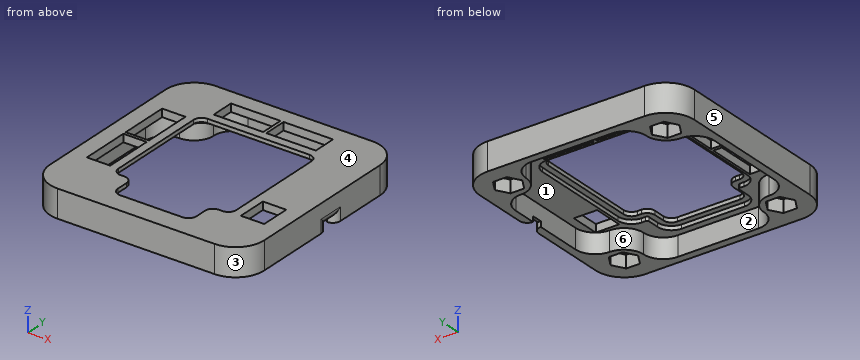
from build123d import *

# Parameters (mm, degrees)
WALL_EXTRUDE_BOSS_START          = 8.64
WALL_EXTRUDE_BOSS_DEPTH          = 7.05
CEILING_EXTRUDE_BOSS_DEPTH       = 2
SCREWS_BLOCKS_EXTRUDE_BOSS_DEPTH = 5.05
SCREWS_BLOCKS_FILLET_R           = 5
NUTS_EXTRUDE_DEPTH               = 3.2
SCREWS_SKETCH_R                  = 2.15
SCREWS_HOOLES_EXTRUDE_DEPTH      = 2.5
CONNECTORS_SKETCH_W              = 12.6
CONNECTORS_SKETCH_H              = 5.95
CONNECTORS_SKETCH_W_2            = 5.95
CONNECTORS_SKETCH_H_2            = 12.6
CONNECTORS_SKETCH_H_3            = 7.6
CONNECTORS_EXTRUDE_DEPTH         = 2.5
SWITCH_SKETCH_W                  = 1.4
SWITCH_SKETCH_H                  = 2.68
SWITCH_EXTRUDE_DEPTH             = 2.5
SWITCH_FILLET_R                  = 2
GLASS_EXTRUDE_DEPTH              = 2.5
GLASS_FIT_EXTRUDE_DEPTH          = 1


with BuildPart() as part:
    # Wall_Sketch → Wall_Extrude_Boss (new body)
    with BuildSketch(Plane.XY.offset(WALL_EXTRUDE_BOSS_START)):
        with BuildLine():
            Line((-52.3, 44.999999897), (-52.29999, 5.00000605))
            ThreePointArc((-52.29999, 5.00000605), (-50.161874571, -0.161870293), (-45, -2.29999))
            Line((-45, -2.29999), (-5.000000575, -2.3))
            ThreePointArc((-5.000000575, -2.3), (0.161879299, -0.161879706), (2.3, 5))
            Line((2.3, 5), (2.3, 45))
            ThreePointArc((2.3, 45), (0.161879503, 50.161879503), (-5, 52.3))
            Line((-5, 52.3), (-45, 52.3))
            ThreePointArc((-45, 52.3), (-50.161879539, 50.161879466), (-52.3, 44.999999897))
        make_face()
        with BuildLine():
            Line((-5, 50.3), (-45, 50.3))
            ThreePointArc((-45, 50.3), (-48.747665967, 48.747665914), (-50.3, 44.999999925))
            Line((-50.3, 44.999999925), (-50.29999, 5.00000655))
            ThreePointArc((-50.29999, 5.00000655), (-48.747661185, 1.252343447), (-45, -0.29999))
            Line((-45, -0.29999), (-5.000000075, -0.3))
            ThreePointArc((-5.000000075, -0.3), (-1.252334086, 1.252334033), (0.3, 5))
            Line((0.3, 5), (0.3, 45))
            ThreePointArc((0.3, 45), (-1.25233406, 48.74766594), (-5, 50.3))
        make_face(mode=Mode.SUBTRACT)
    extrude(amount=-WALL_EXTRUDE_BOSS_DEPTH)

    # Ceiling_Sketch → Ceiling_Extrude_Boss (add)
    with BuildSketch(Plane.XY.offset(8.64)):
        with BuildLine():
            Line((-45, -0.29999), (-5.000000075, -0.3))
            ThreePointArc((-5.000000075, -0.3), (-1.252334086, 1.252334033), (0.3, 5))
            Line((0.3, 5), (0.3, 45))
            ThreePointArc((0.3, 45), (-1.25233406, 48.74766594), (-5, 50.3))
            Line((-5, 50.3), (-45, 50.3))
            ThreePointArc((-45, 50.3), (-48.747665967, 48.747665914), (-50.3, 44.999999925))
            Line((-50.3, 44.999999925), (-50.29999, 5.00000655))
            ThreePointArc((-50.29999, 5.00000655), (-48.747661185, 1.252343447), (-45, -0.29999))
        make_face()
    extrude(amount=-CEILING_EXTRUDE_BOSS_DEPTH)


with BuildPart() as screws_blocks_extrude_boss_tool:
    # Screws_Blocks_Sketch → Screws_Blocks_Extrude_Boss (new body)
    with BuildSketch(Plane(origin=(0, 0, 6.64), x_dir=(-1, 0, 0), z_dir=(0, 0, -1))):
        with BuildLine():
            Line((9.7, -0.299998825), (4.7, -0.299998825))
            ThreePointArc((4.7, -0.299998825), (1.164466094, 1.164467269), (-0.3, 4.700001175))
            Line((-0.3, 4.700001175), (-0.3, 9.700001175))
            Line((-0.3, 9.700001175), (9.7, 9.700001175))
            Line((9.7, 9.700001175), (9.7, -0.299998825))
        make_face()
        with BuildLine():
            Line((9.7, 50.3), (4.7, 50.3))
            ThreePointArc((4.7, 50.3), (1.164466094, 48.835533906), (-0.3, 45.3))
            Line((-0.3, 45.3), (-0.3, 40.3))
            Line((-0.3, 40.3), (9.7, 40.3))
            Line((9.7, 40.3), (9.7, 50.3))
        make_face()
        with BuildLine():
            Line((40.299998825, 50.3), (45.299998825, 50.3))
            ThreePointArc((45.299998825, 50.3), (48.835532731, 48.835533906), (50.299998825, 45.3))
            Line((50.299998825, 45.3), (50.299998825, 40.3))
            Line((50.299998825, 40.3), (40.299998825, 40.3))
            Line((40.299998825, 40.3), (40.299998825, 50.3))
        make_face()
        with BuildLine():
            Line((40.299991175, -0.299991175), (45.299991175, -0.299991175))
            ThreePointArc((45.299991175, -0.299991175), (48.835525081, 1.164474919), (50.299991175, 4.700008825))
            Line((50.299991175, 4.700008825), (50.299991175, 9.700008825))
            Line((50.299991175, 9.700008825), (40.299991175, 9.700008825))
            Line((40.299991175, 9.700008825), (40.299991175, -0.299991175))
        make_face()
    extrude(amount=SCREWS_BLOCKS_EXTRUDE_BOSS_DEPTH)


with BuildPart() as part_1:
    add(part.part)


with BuildPart() as part_2:
    # Screws_Blocks_Extrude_Boss: joined with screws_blocks_extrude_boss_tool
    add(part_1.part.fuse(screws_blocks_extrude_boss_tool.part, tol=0.00001))

    # Screws_Blocks_Fillet
    screws_blocks_fillet_edges = [part_2.edges().sort_by_distance(p)[0] for p in [
        (-40.299998825, 50.3, 4.115),
        (-50.299998825, 40.3, 4.115),
        (-40.299998825, 40.3, 4.115),
        (-9.7, 50.3, 4.115),
        (-9.7, 40.3, 4.115),
        (0.3, 40.3, 4.115),
        (0.3, 9.700001175, 4.115),
        (-9.7, 9.700001175, 4.115),
        (-9.7, -0.299998825, 4.115),
        (-40.299991175, -0.299991175, 4.115),
        (-40.299991175, 9.700008825, 4.115),
        (-50.299991175, 9.700008825, 4.115),
    ]]
    fillet(screws_blocks_fillet_edges, radius=SCREWS_BLOCKS_FILLET_R - 0.0001)  # a hair under: the kernel refuses the full size

    # Nuts_Sketch → Nuts_Extrude (cut)
    with BuildSketch(Plane(origin=(0, 0, 1.59), x_dir=(-1, 0, 0), z_dir=(0, 0, -1))):
        Polygon((1.500002453, 44.995856332), (3.253589748, 41.966841377), (6.753587296, 41.970985045), (8.499997547, 45.004143668), (6.746410252, 48.033158623), (3.246412704, 48.029014955), align=None)
        Polygon((41.5, 45), (43.25, 41.968911087), (46.75, 41.968911087), (48.5, 45), (46.75, 48.031088913), (43.25, 48.031088913), align=None)
        Polygon((41.5, 5), (43.25, 1.968911087), (46.75, 1.968911087), (48.5, 5), (46.75, 8.031088913), (43.25, 8.031088913), align=None)
        Polygon((8.49998026, 4.988245077), (6.760170192, 8.025194356), (3.260189932, 8.03694928), (1.50001974, 5.011754923), (3.239829808, 1.974805644), (6.739810068, 1.96305072), align=None)
    extrude(amount=-NUTS_EXTRUDE_DEPTH, mode=Mode.SUBTRACT)

    # Screws_Sketch → Screws_Hooles_Extrude (cut)
    with BuildSketch(Plane(origin=(0, 0, 4.79), x_dir=(-1, 0, 0), z_dir=(0, 0, -1))):
        with Locations((5, 45)):
            Circle(SCREWS_SKETCH_R)
        with Locations((45, 45)):
            Circle(SCREWS_SKETCH_R)
        with Locations((45, 5)):
            Circle(SCREWS_SKETCH_R)
        with Locations((5, 5)):
            Circle(SCREWS_SKETCH_R)
    extrude(amount=-SCREWS_HOOLES_EXTRUDE_DEPTH, mode=Mode.SUBTRACT)

    # Connectors_Sketch → Connectors_Extrude (cut)
    with BuildSketch(Plane.XY.offset(8.64)):
        with Locations((-31.7, 45.175)):
            Rectangle(CONNECTORS_SKETCH_W, CONNECTORS_SKETCH_H)
        with Locations((-18.3, 45.175)):
            Rectangle(CONNECTORS_SKETCH_W, CONNECTORS_SKETCH_H)
        with Locations((-45.075, 31.7)):
            Rectangle(CONNECTORS_SKETCH_W_2, CONNECTORS_SKETCH_H_2)
        with Locations((-45.075, 18.3)):
            Rectangle(CONNECTORS_SKETCH_W_2, CONNECTORS_SKETCH_H_2)
        with Locations((-4.825, 14.4)):
            Rectangle(CONNECTORS_SKETCH_W_2, CONNECTORS_SKETCH_H_3)
    extrude(amount=-CONNECTORS_EXTRUDE_DEPTH, mode=Mode.SUBTRACT)

    # Switch_Sketch → Switch_Extrude (cut)
    with BuildSketch(Plane(origin=(2.3, 0, 0), x_dir=(0, 0, -1), z_dir=(1, 0, 0))):
        with Locations((-2.24, 28.01)):
            Rectangle(SWITCH_SKETCH_W, SWITCH_SKETCH_H)
    extrude(amount=-SWITCH_EXTRUDE_DEPTH, mode=Mode.SUBTRACT)

    # Switch_Fillet
    switch_fillet_edges = [part_2.edges().sort_by_distance(p)[0] for p in [
        (2.3, 28.01, 2.94),
        (2.3, 29.35, 2.265),
        (2.3, 26.67, 2.265),
    ]]
    fillet(switch_fillet_edges, radius=SWITCH_FILLET_R - 0.0001)  # a hair under: the kernel refuses the full size

    # Glass_Sketch → Glass_Extrude (cut)
    with BuildSketch(Plane(origin=(0, 0, 6.64), x_dir=(-1, 0, 0), z_dir=(0, 0, -1))):
        with BuildLine():
            Line((34.9999975, 8), (34.9999975, 5))
            ThreePointArc((34.9999975, 5), (34.414211062, 3.585786438), (32.9999975, 3))
            Line((32.9999975, 3), (16.9999975, 3))
            ThreePointArc((16.9999975, 3), (15.585783938, 3.585786438), (14.9999975, 5))
            Line((14.9999975, 5), (14.9999975, 8))
            ThreePointArc((14.9999975, 8), (14.414211062, 9.414213562), (12.9999975, 10))
            Line((12.9999975, 10), (11.9999975, 10))
            ThreePointArc((11.9999975, 10), (10.585783938, 10.585786438), (9.9999975, 12))
            Line((9.9999975, 12), (9.9999975, 38))
            ThreePointArc((9.9999975, 38), (10.585783938, 39.414213562), (11.9999975, 40))
            Line((11.9999975, 40), (37.9999975, 40))
            ThreePointArc((37.9999975, 40), (39.414211062, 39.414213562), (39.9999975, 38))
            Line((39.9999975, 38), (39.9999975, 12))
            ThreePointArc((39.9999975, 12), (39.414211062, 10.585786438), (37.9999975, 10))
            Line((37.9999975, 10), (36.9999975, 10))
            ThreePointArc((36.9999975, 10), (35.585783938, 9.414213562), (34.9999975, 8))
        make_face()
    extrude(amount=-GLASS_EXTRUDE_DEPTH, mode=Mode.SUBTRACT)

    # Glass_Fit_Sketch → Glass_Fit_Extrude (cut)
    with BuildSketch(Plane(origin=(0, 0, 6.64), x_dir=(-1, 0, 0), z_dir=(0, 0, -1))):
        with BuildLine():
            Line((36.9999975, 8.5), (37.9999975, 8.5))
            ThreePointArc((37.9999975, 8.5), (40.474871234, 9.525126266), (41.4999975, 12))
            Line((41.4999975, 12), (41.4999975, 38))
            ThreePointArc((41.4999975, 38), (40.474871234, 40.474873734), (37.9999975, 41.5))
            Line((37.9999975, 41.5), (11.9999975, 41.5))
            ThreePointArc((11.9999975, 41.5), (9.525123766, 40.474873734), (8.4999975, 38))
            Line((8.4999975, 38), (8.4999975, 12))
            ThreePointArc((8.4999975, 12), (9.525123766, 9.525126266), (11.9999975, 8.5))
            Line((11.9999975, 8.5), (12.9999975, 8.5))
            ThreePointArc((12.9999975, 8.5), (13.353550891, 8.353553391), (13.4999975, 8))
            Line((13.4999975, 8), (13.4999975, 5))
            ThreePointArc((13.4999975, 5), (14.525123766, 2.525126266), (16.9999975, 1.5))
            Line((16.9999975, 1.5), (32.9999975, 1.5))
            ThreePointArc((32.9999975, 1.5), (35.474871234, 2.525126266), (36.4999975, 5))
            Line((36.4999975, 5), (36.4999975, 8))
            ThreePointArc((36.4999975, 8), (36.646444109, 8.353553391), (36.9999975, 8.5))
        make_face()
    extrude(amount=-GLASS_FIT_EXTRUDE_DEPTH, mode=Mode.SUBTRACT)


solid = part_2.part
The model under review builds one solid part; all positions refer to its coordinate system, in mm. Face numbers are marked on the shaded views. A direction names the side the tool comes from. Give positions to 0.01 mm unless a question says otherwise; leave off trailing zeros. Write each loop counter-clockwise with the first axis right and the second up, starting at its lowest first coordinate (ties: lowest second). Pieces come first, ordered by that corner, then holes.
1. For P1, Ø3, axis at x = -45.5, y = 5, coming from the -Z side; P2, Ø0.6, axis at y = 46.5, z = 8, coming from the -X side; P3, Ø5, axis at x = -5, y = 45, coming from the -Z side, all flat-tipped, find the tip position at first contact; note any pin that passes through.
2. Tool access review of the marked faces 5 and 6: name each direction out of +Z, -Z, +X, -X, +Y, -Y from which nothing blocks a thin tool from reaching the whole face with its end or side.
3. Add section A-A, the plane y = 20. Write out the cut boundary in (x, z), plus the area to 3 significant figures.
4. Draft analysis for pull direction Y (two halves, no side actions). For the marked faces 1, 2, 3 and 4, state which applies: +Y half, -Y half, draft (parallel to the pull), parting line (faces both ways), or undercut.
5. Wall thickness on L1, parallel to Y at x = -20, z = 7; L2, parallel to X at y = 34, z = 7.75; L3, parallel to Y at x = -5, z = 6.4: over which ranges is each line inside the solid? List them lowest first.
Worked answers:
1. P1: stops at z = 7.29
1. P2: stops at x = -52.2
1. P3: stops at z = 4.79
2. face 5: +Z, -Z, -X, +Y, -Y
2. face 6: -Z
3. outline: (-52.3, 1.59) - (-50.3, 1.59) - (-50.3, 6.64) - (-48.05, 6.64) - (-48.05, 8.64) - (-52.3, 8.64) - close; (-42.1, 6.64) - (-41.5, 6.64) - (-41.5, 7.64) - (-40, 7.64) - (-40, 8.64) - (-42.1, 8.64) - close; (-10, 7.64) - (-8.5, 7.64) - (-8.5, 6.64) - (0.3, 6.64) - (0.3, 1.59) - (2.3, 1.59) - (2.3, 8.64) - (-10, 8.64) - close
3. area: 54.5 mm2
4. face 1: undercut
4. face 2: undercut
4. face 3: -Y half
4. face 4: draft
5. L1: y = -2.3 to 1.5, 41.5 to 42.2, 48.15 to 52.3
5. L2: x = -52.3 to -48.05, -42.1 to -40, -10 to 2.3
5. L3: y = -2.3 to 2.85, 7.15 to 9.69, 40.31 to 42.85, 47.15 to 52.3
